The drawing under review shows one solid part. Ordinate dimensions are in mm from its lowest x, y, z. A direction names the side the tool comes from. Coordinates: 2 decimals unless noted, no trailing zeros. Write each loop counter-clockwise with the first axis right and the second up, starting at its lowest first coordinate (ties: lowest second). Pieces come first, ordered by that corner, then holes.
1) For the marked faces 1, 2, 3, 4 and 5, list the 3-axis set-ups (+Z, -Z, +X, -X, +Y, -Y) from which the entire face can be reached by the end or side of a thin tool; tool diameter is ignored.
2) To check wall thickness, follow line 1 along Z through (x, y) = (25, 29.05); line 2 along X through (y, z) = (16, 49); line 3 along Z through (x, y) = (28, 29) (1 decimal). State the ranges of each line that lie inside material, in increasing order.
3) Mouldability with a two-part tool opening along Z and no side actions: class the marked faces 6, 7 and 8 as pulls with the +Z half, pulls with the -Z half, needs draft (parallel to the pull), parting line crosses it, or undercut.
4) We need section A-A on x = 25. Write out the cut boundary in (y, z).
5) Insertion check: P1, Ø7.5, axis at x = 23.5, z = 45.5, coming from the +Y side; P2, Ø13, axis at x = 14.5, z = 30.5, coming from the +Y side; P3, Ø10, axis at y = 42.5, z = 19, coming from the -X side; P4, Ø13, axis at x = 13, y = 24, coming from the -Z side. Each pin has a flat end and moves straight along its axis. Give the tip position at first contact, or say it passes through.
6) We need section D-D on z = 21. Write out the cut boundary in (x, y).
7) We need section B-B on y = 10.5. Write out the cut boundary in (x, z), then the cut area to 3 significant figures.
8) We need section C-C on z = 49. Write out the cut boundary in (x, y).
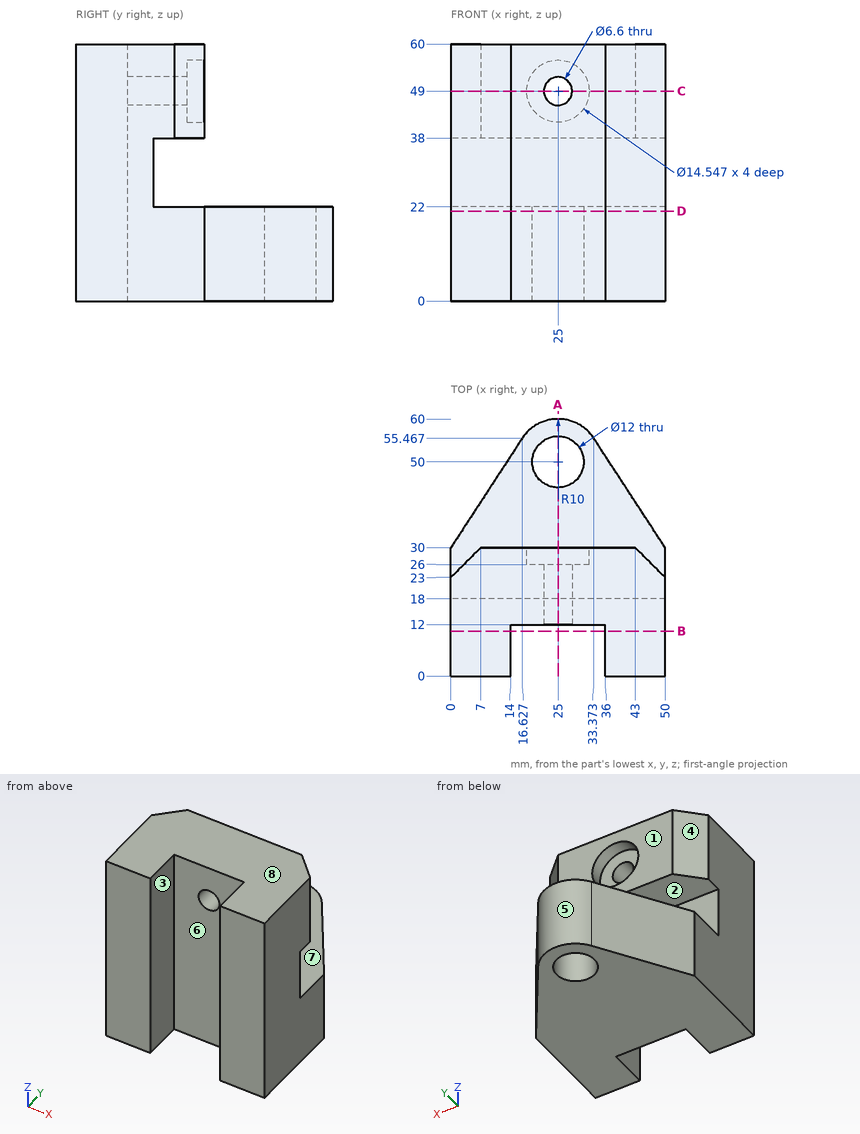
Result:
1. face 1: +Z, +X, -X, +Y
1. face 2: +X, -X, +Y
1. face 3: +Z, -Z, -Y
1. face 4: +Z, -X, +Y
1. face 5: +Z, -Z, +Y
2. line 1: z = 0 to 22, 38 to 41.73, 56.27 to 60
2. line 2: x = 0 to 21.7, 28.3 to 50
2. line 3: z = 0 to 22, 38 to 42.4, 55.6 to 60
3. face 6: needs draft
3. face 7: undercut
3. face 8: pulls with the +Z half
4. outline: (12, 0) - (44, 0) - (44, 22) - (18, 22) - (18, 38) - (30, 38) - (30, 41.73) - (26, 41.73) - (26, 45.7) - (12, 45.7) - close; (12, 52.3) - (26, 52.3) - (26, 56.27) - (30, 56.27) - (30, 60) - (12, 60) - close; (56, 0) - (60, 0) - (60, 22) - (56, 22) - close
5. P1: stops at y = 30
5. P2: stops at y = 18
5. P3: stops at x = 4.9
5. P4: stops at z = 0
6. outline: (0, 0) - (14, 0) - (14, 12) - (36, 12) - (36, 0) - (50, 0) - (50, 30) - (33.37, 55.47) arc R10 ccw to (16.63, 55.47) - (0, 30) - close; hole circle Ø12 at (25, 50)
7. outline: (0, 0) - (14, 0) - (14, 60) - (0, 60) - close; (36, 0) - (50, 0) - (50, 60) - (36, 60) - close
7. area: 1,680 mm2
8. outline: (0, 0) - (14, 0) - (14, 12) - (21.7, 12) - (21.7, 26) - (17.73, 26) - (17.73, 30) - (7, 30) - (0, 23) - close; (28.3, 12) - (36, 12) - (36, 0) - (50, 0) - (50, 23) - (43, 30) - (32.27, 30) - (32.27, 26) - (28.3, 26) - close
